from build123d import *

# Parameters (mm, degrees)
SKETCH1_W           = 8.509
SKETCH1_H           = 8.509
BOSS_EXTRUDE1_DEPTH = 8.509
SKETCH2_W           = 3.9878
SKETCH2_H           = 3.9878
BOSS_EXTRUDE2_DEPTH = 5.6896
SKETCH3_W           = 0.508
SKETCH3_H           = 0.4064
BOSS_EXTRUDE3_DEPTH = 3.5052


with BuildPart() as part:
    # Sketch1 → Boss-Extrude1 (new body)
    with BuildSketch(Plane(origin=(0, 0, 0), x_dir=(1, 0, 0), z_dir=(0, 1, 0))):
        with Locations((4.2545, 4.2545)):
            Rectangle(SKETCH1_W, SKETCH1_H)
    extrude(amount=BOSS_EXTRUDE1_DEPTH)

    # Sketch2 → Boss-Extrude2 (add)
    with BuildSketch(Plane(origin=(0, 8.509, 0), x_dir=(1, 0, 0), z_dir=(0, 1, 0))):
        with Locations((4.2545, 4.2545)):
            Rectangle(SKETCH2_W, SKETCH2_H)
    extrude(amount=BOSS_EXTRUDE2_DEPTH)

    # Sketch3 → Boss-Extrude3 (add)
    with BuildSketch(Plane.XZ):
        with Locations((1.7018, -1.5494)):
            Rectangle(SKETCH3_W, SKETCH3_H)
        with Locations((1.7018, -6.8834)):
            Rectangle(SKETCH3_W, SKETCH3_H)
        with Locations((4.2418, -6.8834)):
            Rectangle(SKETCH3_W, SKETCH3_H)
        with Locations((6.7818, -6.8834)):
            Rectangle(SKETCH3_W, SKETCH3_H)
        with Locations((4.2418, -1.5494)):
            Rectangle(SKETCH3_W, SKETCH3_H)
        with Locations((6.7818, -1.5494)):
            Rectangle(SKETCH3_W, SKETCH3_H)
    extrude(amount=BOSS_EXTRUDE3_DEPTH)


solid = part.part
Work out the finished part from the listing and answer in its coordinate system (mm). A direction names the side the tool comes from. Give positions to 0.01 mm unless a question says otherwise; leave off trailing zeros. Loops run counter-clockwise (first coordinate to the right, second up) from the corner with the lowest first, then second, coordinate; pieces in that order, holes last. Notation, with made-up numbers: (-14, 78.5) - (38, 78.5) arc R12 cw to (38, 92.5) - close; hole circle Ø5 at (88.5, 12.25). An arc over 180 degrees is marked (long way). Answer in a Markdown table with one row per item.
(1) Consider L1, parallel to X at y = -2.5, z = -1.5; L2, parallel to Y at x = 8, z = -6.5; L3, parallel to Y at x = 4.75, z = -4.25. Determine where each line is inside the solid, lowest interval first. Write a range as [from, to].
Results list:
| item | result |
|---|---|
| L1 | x = [1.45, 1.96], [3.99, 4.5], [6.53, 7.04] |
| L2 | y = [0, 8.51] |
| L3 | y = [0, 14.2] |
(2) Section B-B (z = -3) is taken. Give the vertices of the cut face in (x, y), and give its area (3 significant figures).
Results list:
| item | result |
|---|---|
| outline | (0, 0) - (8.51, 0) - (8.51, 8.51) - (6.25, 8.51) - (6.25, 14.2) - (2.26, 14.2) - (2.26, 8.51) - (0, 8.51) - close |
| area | 95.1 mm² |
(3) Section A-A (x = 4.25) is taken. Give the vertices of the cut face in (y, z), and give its area (3 significant figures).
Results list:
| item | result |
|---|---|
| outline | (-3.51, -7.09) - (0, -7.09) - (0, -8.51) - (8.51, -8.51) - (8.51, -6.25) - (14.2, -6.25) - (14.2, -2.26) - (8.51, -2.26) - (8.51, 0) - (0, 0) - (0, -1.35) - (-3.51, -1.35) - (-3.51, -1.75) - (0, -1.75) - (0, -6.68) - (-3.51, -6.68) - close |
| area | 97.9 mm² |
(4) Section D-D (x = 2.5) is taken. Give the vertices of the cut face in (y, z), and give its area (3 significant figures).
Results list:
| item | result |
|---|---|
| outline | (0, -8.51) - (8.51, -8.51) - (8.51, -6.25) - (14.2, -6.25) - (14.2, -2.26) - (8.51, -2.26) - (8.51, 0) - (0, 0) - close |
| area | 95.1 mm² |
(5) Section C-C (y = 11.25) is taken. Give the vertices of the cut face in (x, z).
Results list:
| item | result |
|---|---|
| outline | (2.26, -6.25) - (6.25, -6.25) - (6.25, -2.26) - (2.26, -2.26) - close |
(6) For a pull along Z with two mould halves and no side action, classify faces 5 (the face through (8.509, 4, -4)), 6 (the face through (4, 0, -4)), 7 (the face through (4, 11, -2.261)) as pulls with the +Z half, pulls with the -Z half, needs draft (parallel to the pull), parting line crosses it, or undercut.
Results list:
| item | result |
|---|---|
| face 5 | needs draft |
| face 6 | undercut |
| face 7 | pulls with the +Z half |
(7) Flat-ended cylindrical pins translate along their axes: pin 1 Ø0.6 at (x, y) = (1.5, -2) entering from +Z; pin 2 Ø0.6 at (x, y) = (7, -2) entering from -Z; pin 3 Ø1.5 at (x, y) = (4, 11) entering from -Z. Find the tip coordinate at first contact, or state that the pin passes through.
Results list:
| item | result |
|---|---|
| pin 1 | stops at z = -1.35 |
| pin 2 | stops at z = -7.09 |
| pin 3 | stops at z = -6.25 |
(8) A tool of negligible diameter and unlimited length cuts with its end or side. For faces 1 (the face through (4, 14.199, -4)), 2 (the face through (4, 11, -6.248)), 3 (the face through (2.261, 11, -4)), 4 (the face through (6.248, 11, -4)), from which of +Z, -Z, +X, -X, +Y, -Y can it reach the whole face along a straight path? Write none if from no direction.
Results list:
| item | result |
|---|---|
| face 1 | +Z, -Z, +X, -X, +Y |
| face 2 | -Z, +X, -X, +Y |
| face 3 | +Z, -Z, -X, +Y |
| face 4 | +Z, -Z, +X, +Y |
